Work out the finished part from the listing and answer in its coordinate system (mm). A direction names the side the tool comes from. Coordinates: 2 decimals unless noted, no trailing zeros. Order: outer loops, then holes, each group sorted by start corner. A loop starts at its lowest first (then second) coordinate and runs counter-clockwise, first axis right, second up.
```python
from build123d import *

# Parameters (mm, degrees)
F0_R     = 15
F1_DEPTH = 5
F2_R     = 16
F2_R_2   = 15
F3_DEPTH = 2.5
F5_DEPTH = 2.5
F7_DEPTH = 2.5
F9_D     = 1.5


with BuildPart() as f1:
    # F0 (on Front) → F1 (new body)
    with BuildSketch(Plane.XZ):
        with BuildLine():
            Line((-18.939282, -6), (-16.439282, -6))
            ThreePointArc((-16.439282, -6), (0, -17.5), (16.439282, -6))
            Line((16.439282, -6), (18.939282, -6))
            Line((18.939282, -6), (18.939282, 6))
            Line((18.939282, 6), (16.439282, 6))
            ThreePointArc((16.439282, 6), (0, 17.5), (-16.439282, 6))
            Line((-16.439282, 6), (-18.939282, 6))
            Line((-18.939282, 6), (-18.939282, -6))
        make_face()
        Circle(F0_R, mode=Mode.SUBTRACT)
    extrude(amount=F1_DEPTH)

    # F2 (on face) → F3 (cut)
    with BuildSketch(Plane.XZ.offset(5)):
        Circle(F2_R)
        Circle(F2_R_2, mode=Mode.SUBTRACT)
    extrude(amount=-F3_DEPTH, mode=Mode.SUBTRACT)

    # F4 (on face) → F5 (cut)
    with BuildSketch(Plane(origin=(-18.939282, 0, 0), x_dir=(0, -1, 0), z_dir=(-1, 0, 0))):
        with BuildLine():
            Line((5, -3.1), (5, 3.1))
            ThreePointArc((5, 3.1), (1.9, 0), (5, -3.1))
        make_face()
    extrude(amount=-F5_DEPTH, mode=Mode.SUBTRACT)

    # F6 (on face) → F7 (cut)
    with BuildSketch(Plane.YZ.offset(18.939282)):
        with BuildLine():
            ThreePointArc((-5, -3.1), (-1.9, 0), (-5, 3.1))
            Line((-5, 3.1), (-5, -3.1))
        make_face()
    extrude(amount=-F7_DEPTH, mode=Mode.SUBTRACT)

    # F9 (through all)
    with Locations(Plane(origin=(0, 0, 0), x_dir=(1, 0, 0), z_dir=(0, 1, 0))):
        with Locations((-17, 4.5), (-17, -4.5), (17, -4.5), (17, 4.5)):
            Hole(F9_D / 2)


solid = f1.part
```
1. The mould has two halves that part along X. Classify faces 4 (the flat face through (16.439, -4, 0)), 5 (the cylindrical face through (0.299, -2.465, 17.497)), 6 (the cylindrical face through (-16.405, -2.535, -4.044)), 7 (the cylindrical face through (17.595, -2.535, 4.956)): released by +X, released by -X, zero draft, split by the parting line, or undercut.
2. The part is cut by section D-D (x = 9.5). Determine the outline of the cut face in (y, z), plus the area to 3 significant figures.
3. The part is cut by section B-B (y = -1.1). Determine the outline of the cut face in (x, z).
4. The part is cut by section A-A (x = 17). Determine the outline of the cut face in (y, z).
5. Flat-ended cylindrical pins translate along their axes: pin 1 (1.6 mm diameter, centred on y = -3, z = -1, fed in from +X); pin 2 (1.5 mm diameter, centred on x = -9.5, y = -3, fed in from +Z); pin 3 (0.8 mm diameter, centred on x = -18.5, y = -3.5, fed in from +Z). Find the tip coordinate at first contact, or state that the pin passes through.
6. The part is cut by section C-C (z = 4.5). Determine the outline of the cut face in (x, y).
7. Consider probe 1 along X at (y, z) = (-2.2, 4); probe 2 along Z at (x, y) = (17, -2.5); probe 3 along X at (y, z) = (-3.8, 4.5). Determine where each line is inside the solid, lowest interval first.
8. For faces 1 (the flat face through (-16.439, -4, 0)), 2 (the flat face through (18, -2, -6)), 3 (the flat face through (18, -2, 6)), determine the directions among +Z, -Z, +X, -X, +Y, -Y from which every point of the face is accessible in a straight line to the end or side of a thin tool.
Worked out:
1. face 4: released by +X
1. face 5: split by the parting line
1. face 6: undercut
1. face 7: undercut
2. outline: (-5, -14.7) - (0, -14.7) - (0, -11.61) - (-2.5, -11.61) - (-2.5, -12.87) - (-5, -12.87) - close; (-5, 12.87) - (-2.5, 12.87) - (-2.5, 11.61) - (0, 11.61) - (0, 14.7) - (-5, 14.7) - close
2. area: 24.6 mm2
3. outline: (-18.94, -6) - (-16.44, -6) arc R17.5 ccw to (16.44, -6) - (18.94, -6) - (18.94, 6) - (16.44, 6) arc R17.5 ccw to (-16.44, 6) - (-18.94, 6) - close; hole circle Ø1.5 at (-17, -4.5); hole circle Ø1.5 at (-17, 4.5); hole circle Ø30 at (0, 0); hole circle Ø1.5 at (17, -4.5); hole circle Ø1.5 at (17, 4.5)
4. outline: (-5, -6) - (0, -6) - (0, -5.25) - (-5, -5.25) - close; (-5, -3.75) - (0, -3.75) - (0, 3.75) - (-5, 3.75) - (-5, 3.1) arc R3.1 cw to (-5, -3.1) - close; (-5, 5.25) - (0, 5.25) - (0, 6) - (-5, 6) - close
5. pin 1: stops at x = 16.44
5. pin 2: stops at z = 15.16
5. pin 3: stops at z = 6
6. outline: (-18.94, -5) - (-17.75, -5) - (-17.75, 0) - (-18.94, 0) - close; (-16.25, -5) - (-15.35, -5) - (-15.35, -2.5) - (-14.31, -2.5) - (-14.31, 0) - (-16.25, 0) - close; (14.31, -2.5) - (15.35, -2.5) - (15.35, -5) - (16.25, -5) - (16.25, 0) - (14.31, 0) - close; (17.75, -5) - (18.94, -5) - (18.94, 0) - (17.75, 0) - close
7. probe 1: x = -18.94 to -17.56, -16.44 to -14.46, 14.46 to 16.44, 17.56 to 18.94
7. probe 2: z = -6 to -5.25, -3.75 to -1.83, 1.83 to 3.75, 5.25 to 6
7. probe 3: x = -18.94 to -17.75, -16.25 to -15.35, 15.35 to 16.25, 17.75 to 18.94
8. face 1: -X, -Y
8. face 2: -Z, +X, +Y, -Y
8. face 3: +Z, +X, +Y, -Y
